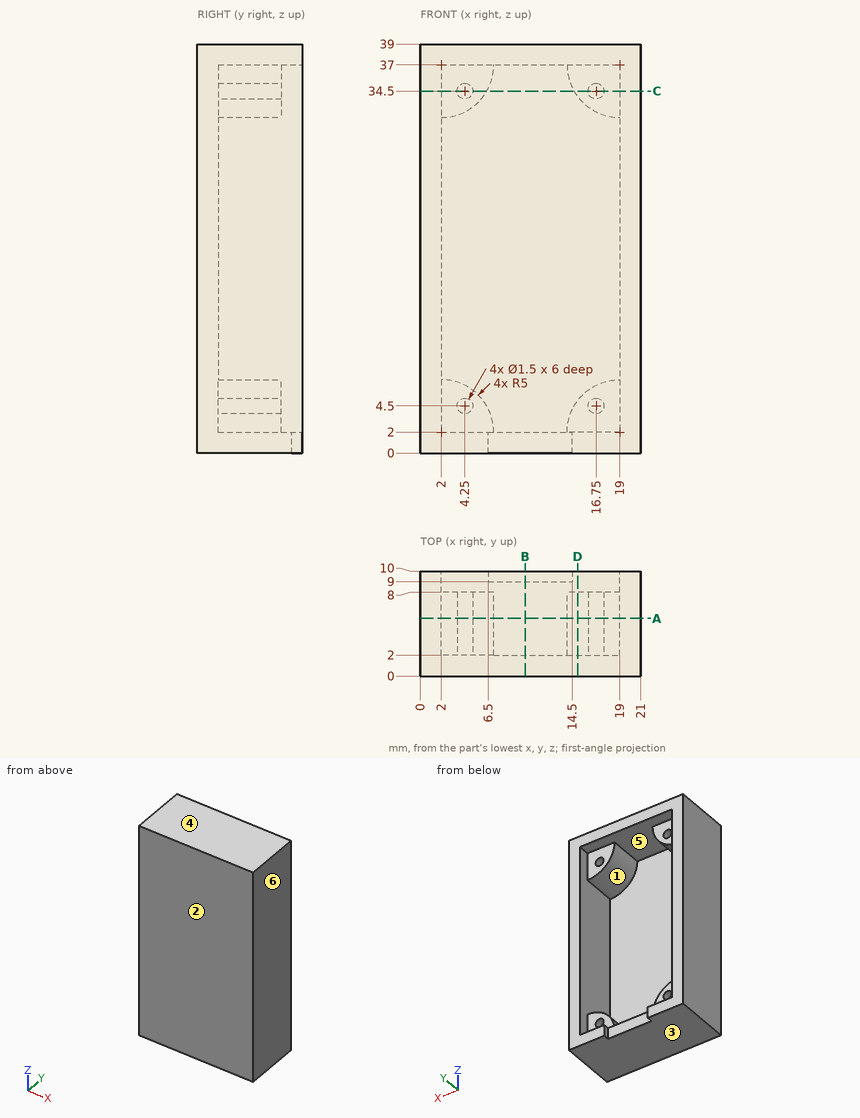
Answer from the drawing. Dimensions are ordinates in mm from the lowest x, y and z of the part. A direction names the side the tool comes from. Round coordinates to 2 decimals unless told otherwise and drop trailing zeros. Loops run counter-clockwise (first coordinate to the right, second up) from the corner with the lowest first, then second, coordinate; pieces in that order, holes last.
(1) The part is cut by section C-C, the plane z = 34.5. Give the vertices of the cut face in (x, y), and give its area (3 significant figures).
Computed values:
outline: (0, 0) - (21, 0) - (21, 10) - (19, 10) - (19, 8) - (17.5, 8) - (17.5, 2) - (16, 2) - (16, 8) - (14.67, 8) - (14.67, 2) - (6.33, 2) - (6.33, 8) - (5, 8) - (5, 2) - (3.5, 2) - (3.5, 8) - (2, 8) - (2, 10) - (0, 10) - close
area: 108 mm2
(2) The mould has two halves that part along Z. Classify the marked faces 3, 4, 5 and 6: pulls with the +Z half, pulls with the -Z half, needs draft (parallel to the pull), parting line crosses it, or undercut.
Computed values:
face 3: pulls with the -Z half
face 4: pulls with the +Z half
face 5: undercut
face 6: needs draft
(3) The part is cut by section B-B, the plane x = 10. Give the vertices of the cut face in (y, z), and give its area (3 significant figures).
Computed values:
outline: (0, 0) - (9, 0) - (9, 2) - (2, 2) - (2, 37) - (10, 37) - (10, 39) - (0, 39) - close
area: 108 mm2
(4) For the marked faces 1 and 2, determine the directions among +Z, -Z, +X, -X, +Y, -Y from which every point of the face is accessible in a straight line to the end or side of a thin tool.
Computed values:
face 1: +Y
face 2: +Z, -Z, +X, -X, -Y
(5) The part is cut by section D-D, the plane x = 15. Give the vertices of the cut face in (y, z), and give its area (3 significant figures).
Computed values:
outline: (0, 0) - (10, 0) - (10, 2) - (8, 2) - (8, 5) - (2, 5) - (2, 34) - (8, 34) - (8, 37) - (10, 37) - (10, 39) - (0, 39) - close
area: 146 mm2
(6) Find the intervals of material crossed by L1, parallel to X at y = 6.3, z = 4.5; L2, parallel to X at y = 8.75, z = 10.5; L3, parallel to Z at x = 7.75, y = 6, in increasing order.
Computed values:
L1: x = 0 to 3.5, 5 to 6.33, 14.67 to 16, 17.5 to 21
L2: x = 0 to 2, 19 to 21
L3: z = 0 to 2, 37 to 39
(7) Each of these flat-tipped pins is pushed along its axis until it touches: P1, Ø8, axis at x = 7, z = 19.5, coming from the +Y side; P2, Ø1.5, axis at x = 2.5, y = 8, coming from the -Z side; P3, Ø0.6, axis at x = 10, z = 1, coming from the +Y side; P4, Ø2.5, axis at x = 4.25, z = 34.5, coming from the +Y side. Where does it stop, or does it pass through?
Computed values:
P1: stops at y = 2
P2: stops at z = 0
P3: stops at y = 9
P4: stops at y = 8
(8) The part is cut by section A-A, the plane y = 5.5. Give the vertices of the cut face in (x, z).
Computed values:
outline: (0, 0) - (21, 0) - (21, 39) - (0, 39) - close; hole (2, 7) arc R5 cw to (7, 2) - (14, 2) arc R5 cw to (19, 7) - (19, 32) arc R5 cw to (14, 37) - (7, 37) arc R5 cw to (2, 32) - close; hole circle Ø1.5 at (4.25, 4.5); hole circle Ø1.5 at (4.25, 34.5); hole circle Ø1.5 at (16.75, 4.5); hole circle Ø1.5 at (16.75, 34.5)
